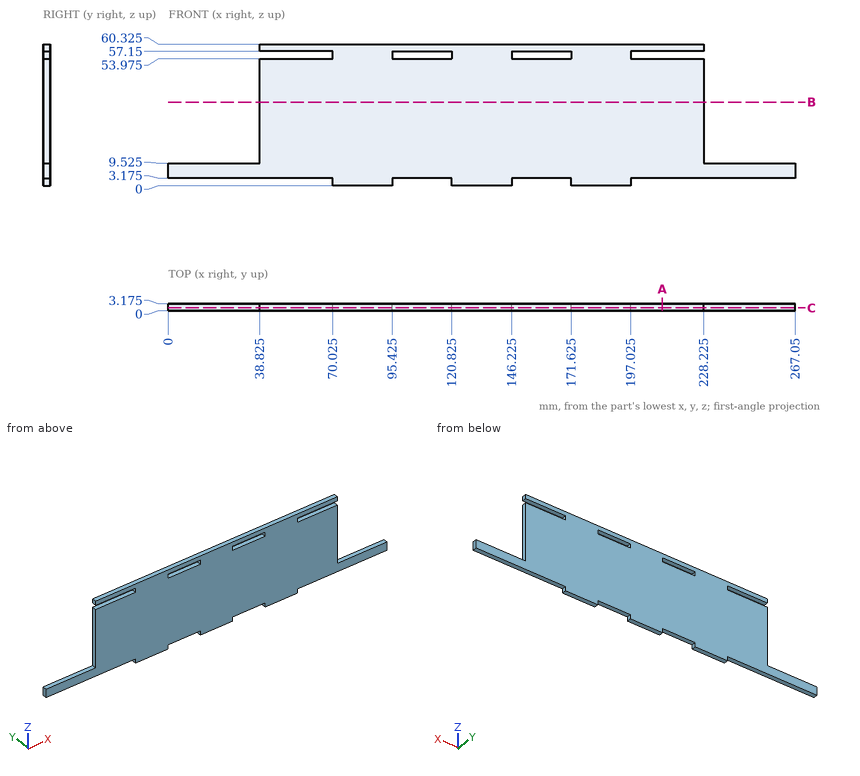
For this review, use the dimensioned drawing (mm, ordinates from the lowest corner) and the shaded views. Coordinates: 2 decimals unless noted, no trailing zeros. Write each loop counter-clockwise with the first axis right and the second up, starting at its lowest first coordinate (ties: lowest second). Pieces come first, ordered by that corner, then holes. Notation, with made-up numbers: (35, 20) - (84, 20) arc R30 cw to (84, 48) - close; hole circle Ø4 at (86, 48.5). An arc over 180 degrees is marked (long way). Answer as a JSON object with one key per item and string values. Group by question number.
1. Add section B-B (z = 35.5). Give the boundary of the cut face in (x, y) (3 decimals).
2. Clearance check with flat-ended pins moving along their axes: pin 1 Ø1 at (x, y) = (11, 2) entering from +Z (3 decimals); pin 2 Ø1 at (y, z) = (1, 56) entering from -X (3 decimals); pin 3 Ø1.6 at (y, z) = (2, 1) entering from +X (3 decimals). State where each tip first meets the part, or that it passes through.
3. To check wall thickness, follow probe 1 along X at (y, z) = (0.85, 54.5) (3 decimals); probe 2 along Z at (x, y) = (65.5, 2.4) (3 decimals); probe 3 along X at (y, z) = (0.3, 28) (3 decimals). State the ranges of each line that lie inside material, in increasing order.
4. Add section A-A (x = 210.5). Give the boundary of the cut face in (y, z) (3 decimals), plus the area to 3 significant figures.
5. Add section C-C (y = 1.3). Give the number of separate pieces and of enclosed holes in the cut face, plus the area to 3 significant figures.
Findings:
{
 "1": {"outline": "(38.825, 0) - (228.225, 0) - (228.225, 3.175) - (38.825, 3.175) - close"},
 "2": {"pin 1": "z = 9.525", "pin 2": "x = 70.025", "pin 3": "x = 197.025"},
 "3": {"probe 1": "70.025 to 95.425, 120.825 to 146.225, 171.625 to 197.025", "probe 2": "3.175 to 53.975, 57.15 to 60.325", "probe 3": "38.825 to 228.225"},
 "4": {"outline": "(0, 3.175) - (3.175, 3.175) - (3.175, 53.975) - (0, 53.975) - close; (0, 57.15) - (3.175, 57.15) - (3.175, 60.325) - (0, 60.325) - close", "area": "171 mm²"},
 "5": {"separate pieces": "1", "enclosed holes": "2", "area": "11,200 mm²"}
}
